Part model, mm, in its own coordinate system. A direction names the side the tool comes from. Coordinates: 2 decimals unless noted, no trailing zeros. Write each loop counter-clockwise with the first axis right and the second up, starting at its lowest first coordinate (ties: lowest second). Pieces come first, ordered by that corner, then holes. Notation, with made-up numbers: (30.25, 1) -> (80.25, 1) arc R21 ccw to (80.25, 20) -> close; hole circle Ø9 at (4, 29.5). An arc over 180 degrees is marked (long way). One line per question, with ' | ' between items. Start each with the question number.
Item 1: Probe probe 1 along Y at (x, z) = (35, -1.45); probe 2 along Y at (x, z) = (-33, -3); probe 3 along X at (y, z) = (8, -3.5). List the from-to ranges inside material, lowest first. Write a range as [from, to].
Item 2: 3-axis set-ups, long thin cutter, end or side, ignore diameter. For faces 1 (the cylindrical face through (13.887, -10.648, 0.986)), 2 (the cylindrical face through (33.054, 18.289, 0.196)), 3 (the cylindrical face through (-45.196, 0.28, 0.289)), 4 (the cylindrical face through (33.054, -18.196, 0.289)), 5 (the cylindrical face through (-23.846, 7.509, -2.028)): which of +Z, -Z, +X, -X, +Y, -Y reach the whole face in a straight line?
Item 3: Saw through at D-D (z = -2.75). List the corners of the cut face in (x, y), and give its area (3 significant figures).
Item 4: Pin check, flat tips, straight feed: pin 1 (4 mm diameter, centred on x = -35, y = 10, fed in from -Z); pin 2 (1.5 mm diameter, centred on x = -15.5, z = 1, fed in from -Y); pin 3 (1 mm diameter, centred on x = 3, z = -2.5, fed in from -Y); pin 4 (3 mm diameter, centred on y = 6.5, z = -0.5, fed in from +X). Stop position of each tip, or through.
Item 5: Saw through at C-C (x = 35). Count the separate pieces of the cut face and the enclosed holes in it, and give its area (3 significant figures).
Item 6: Two-plate mould, pull along Y, no slides. Class faces 6 (the cylindrical face through (-33.439, -18.196, 0.289)), 7 (the cylindrical face through (45.289, 0.28, 0.196)), 8 (the cylindrical face through (33.79, -8.103, -1.042)), 9 (the cylindrical face through (-33.439, 18.196, 0.289)): pulls with the +Y half, pulls with the -Y half, needs draft (parallel to the pull), parting line crosses it, or undercut.
from build123d import *

# Parameters (mm, degrees)
SKETCH1_R            = 30
BOSS_EXTRUDE1_DEPTH  = 2
BOSS_EXTRUDE2_START  = 4
SKETCH2_R            = 30
SKETCH2_R_2          = 25
BOSS_EXTRUDE2_DEPTH  = 4
BOSS_EXTRUDE3_REACH  = 44.849
SKETCH3_W            = 94
SKETCH3_H            = 40
SKETCH4_R            = 25
CUT_EXTRUDE1_DEPTH   = 4
SKETCH5_R            = 17.5
CUT_EXTRUDE2_DEPTH   = 56.901699437
FILLET1_R            = 6
M4_CLEARANCE_HOLE1_D = 4.5


with BuildPart() as part:
    # Sketch1 → Boss-Extrude1 (new body)
    with BuildSketch(Plane.XY):
        Circle(SKETCH1_R)
    extrude(amount=BOSS_EXTRUDE1_DEPTH)

    # Sketch2 → Boss-Extrude2 (add)
    with BuildSketch(Plane(origin=(0, 0, 0), x_dir=(-1, 0, 0), z_dir=(0, 0, -1)).offset(BOSS_EXTRUDE2_START)):
        Circle(SKETCH2_R)
        Circle(SKETCH2_R_2, mode=Mode.SUBTRACT)
    extrude(amount=-BOSS_EXTRUDE2_DEPTH)

    # Boss-Extrude3: up to this face of the body (flat: up to its plane)
    boss_extrude3_end = Plane(part.part.faces().sort_by_distance((0, 0, 2))[0])
    # Sketch3 → Boss-Extrude3 (add, up to the picked face)
    with BuildSketch(Plane(origin=(0, 0, -4), x_dir=(-1, 0, 0), z_dir=(0, 0, -1)), mode=Mode.PRIVATE) as boss_extrude3_sk1:
        Rectangle(SKETCH3_W, SKETCH3_H)
    boss_extrude3_tool1 = split(extrude(boss_extrude3_sk1.sketch, amount=-BOSS_EXTRUDE3_REACH, mode=Mode.PRIVATE), bisect_by=boss_extrude3_end, keep=Keep.BOTH, mode=Mode.PRIVATE)
    add(boss_extrude3_tool1.solids().sort_by(Axis((0, 0, -4), (0, 0, 1)))[0])

    # Sketch4 → Cut-Extrude1 (cut)
    with BuildSketch(Plane(origin=(0, 0, -4), x_dir=(-1, 0, 0), z_dir=(0, 0, -1))):
        Circle(SKETCH4_R)
    extrude(amount=-CUT_EXTRUDE1_DEPTH, mode=Mode.SUBTRACT)

    # Sketch5 → Cut-Extrude2 (cut, through all)
    with BuildSketch(Plane(origin=(0, 0, 0), x_dir=(-1, 0, 0), z_dir=(0, 0, -1))):
        Circle(SKETCH5_R)
    extrude(amount=-CUT_EXTRUDE2_DEPTH, mode=Mode.SUBTRACT)

    # Fillet1
    fillet1_edges = [part.edges().sort_by_distance(p)[0] for p in [
        (47, 0, 2),
        (34.680339887, -20, 2),
        (34.680339887, 20, 2),
        (0, 30, 2),
        (0, -30, 2),
        (-34.680339887, -20, 2),
        (-47, 0, 2),
        (-34.680339887, 20, 2),
    ]]
    fillet(fillet1_edges, radius=FILLET1_R - 0.0001)  # a hair under: the kernel refuses the full size

    # M4 Clearance Hole1 (through all)
    with Locations(Plane.XY.offset(2)):
        with Locations((-35, 10), (-35, -10), (35, 10), (35, -10)):
            Hole(M4_CLEARANCE_HOLE1_D / 2)


solid = part.part
From the geometry:
1) probe 1: [-19.43, -12.25], [-7.75, 7.75], [12.25, 19.43] | probe 2: [-19.92, -11.03], [-8.97, 8.97], [11.03, 19.92] | probe 3: [-46.98, -36.03], [-33.97, -23.69], [23.69, 33.97], [36.03, 46.98]
2) face 1: +Z, -Z | face 2: +Z, +X, +Y | face 3: +Z, -X, +Y, -Y | face 4: +Z, +X, -Y | face 5: -Z
3) outline: (-46.87, -19.87) -> (-22.3, -19.87) arc R29.87 ccw to (22.3, -19.87) -> (46.87, -19.87) -> (46.87, 19.87) -> (22.3, 19.87) arc R29.87 ccw to (-22.3, 19.87) -> (-46.87, 19.87) -> close; hole circle Ø4.5 at (-35, -10); hole circle Ø4.5 at (-35, 10); hole circle Ø50 at (0, 0); hole circle Ø4.5 at (35, -10); hole circle Ø4.5 at (35, 10) | area: 2,320 mm2
4) pin 1: through | pin 2: y = -23.72 | pin 3: y = -29.78 | pin 4: x = 46.66
5) separate pieces: 3 | enclosed holes: 0 | area: 171 mm2
6) face 6: pulls with the -Y half | face 7: needs draft | face 8: undercut | face 9: pulls with the +Y half
